Autodesk Inventor part; units mm, degrees
ref_plane "YZ Plane" through (0, 0, 0) normal (1, 0, 0) x (0, 1, 0)
ref_plane "XZ Plane" through (0, 0, 0) normal (0, 1, 0) x (-1, 0, 0)
ref_plane "XY Plane" through (0, 0, 0) normal (0, 0, 1) x (1, 0, 0)
sketch "Sketch10" plane through (0, 0, 0) normal (1, 0, 0) x (0, 1, 0)
  line L0 (0, 0) -> (175, 0)
  line L1 (350, -175) -> (350, -175)
  line L2 (175, -350) -> (0, -350)
  line L3 (0, -350) -> (0, 0)
  arc A0 (350, -175) -> (175, 0) centre (175, -175) ccw
  arc A1 (175, -350) -> (350, -175) centre (175, -175) ccw
  point P0 (350, -350)
  point P1 (350, 0)
  dimension "d73" = 350
  dimension "d74" = 350
  dimension "d76" = 175
extrude "Extrusion19" add sketch "Sketch10" along normal blind 300
sketch "Sketch11" plane through (300, 0, 0) normal (1, 0, 0) x (0, 0, -1)
  arc A0 (350, 175) -> (0, 175) centre (175, 175) ccw
  circle A1 centre (175, 175) radius 60
  point P0 (0, 0)
  dimension "d79" = 120
extrude "Extrusion20" cut sketch "Sketch11" against normal blind 300
sketch "Sketch12" plane through (0, 0, -350) normal (0, -1, 0) x (1, 0, 0)
  line L0 (300, 0) -> (300, 350)
  line L1 (0, 350) -> (300, 350)
  line L2 (300, 350) -> (300, 0)
  line L3 (300, 0) -> (0, 0)
  line L4 (0, 0) -> (0, 350)
extrude "Extrusion21" add sketch "Sketch12" along normal blind 700
sketch "Sketch13" plane through (300, 0, 0) normal (1, 0, 0) x (0, 0, -1)
  circle A0 centre (175, 175) radius 60
  arc A1 (350, 175) -> (0, 175) centre (175, 175) ccw
  arc A2 (350, 175) -> (0, 175) centre (175, 175) ccw
  line L0 (350, 175) -> (350, 0)
  line L1 (350, 0) -> (0, 0)
  line L2 (0, 0) -> (0, 175)
  circle A3 centre (175, 175) radius 60
extrude "Extrusion22" add sketch "Sketch13" along normal blind 150
properties part number "Molde" material "Aluminum 6061"
Can you work these out from the model? Positions are in its coordinate system, mm. A direction names the side the tool comes from. Give positions to 0.01 mm unless a question says otherwise; leave off trailing zeros. Order: outer loops, then holes, each group sorted by start corner. A loop starts at its lowest first (then second) coordinate and runs counter-clockwise, first axis right, second up. Notation, with made-up numbers: M -36.5,43.25 L 22.5,43.25 A19 cw 22.5,76.25 Z; hole C 73,35.5 d8. An arc over 180 degrees is marked long. Write item = value, one per line. Start each with the question number.
Q1. Suppose I cut it at C-C (y = 187.5). Write out the boundary of the cut face in (x, z).
Q2. Will these pins go through, and if not, where does the flat tip stop? pin 1 Ø2 at (x, z) = (144, -104.5) entering from +Y; pin 2 Ø12 at (y, z) = (-503.5, -207.5) entering from +X; pin 3 Ø10 at (y, z) = (-394, -297.5) entering from -X.
Q3. Suppose I cut it at A-A (z = -175). Write out the boundary of the cut face in (x, y), plus the area to 4 significant figures.
Q4. For faces 1 (the flat face through (450, 100, -173)), 2 (the flat face through (374, 0, -177)), which set-ups out of +Z, -Z, +X, -X, +Y, -Y let a thin tool reach every point of the face, with its end or its side?
Q5. I need wall thicknesses on probe 1 along Y at (x, z) = (94, -175); probe 2 along Y at (x, z) = (351, -175); probe 3 along X at (y, z) = (-565, -86.5). Which ranges of each line are inside material? Lowest first, please. Write a range as [from, to].
Q6. Suppose I cut it at D-D (x = 423.5). Write out the boundary of the cut face in (y, z).
Q7. We'd pull the mould along Z, two halves only. Please class faces 3 (the flat face through (300, -345, -177)), 4 (the flat face through (172, -269, 0)), 5 (the cylindrical face through (221.85, 134.449, -130.778)): pulls with the +Z half, pulls with the -Z half, needs draft (parallel to the pull), parting line crosses it, or undercut.
Q8. Suppose I cut it at B-B (x = 36). Write out the boundary of the cut face in (y, z), plus the area to 3 significant figures.
Check result:
q1.outline = M 0,-349.55 L 450,-349.55 L 450,-233.68 L 0,-233.68 Z; M 0,-116.32 L 450,-116.32 L 450,-0.45 L 0,-0.45 Z
q2.pin_1 = 335.61
q2.pin_2 = 300
q2.pin_3 = 0
q3.outline = M 0,-700 L 300,-700 L 300,0 L 450,0 L 450,115 L 0,115 Z; M 0,235 L 450,235 L 450,350 L 0,350 Z
q3.area = 313,500 mm2
q4.face_1 = +Z, -Z, +X, +Y, -Y
q4.face_2 = +Z, -Z, +X, -Y
q5.probe_1 = [-700, 115], [235, 350]
q5.probe_2 = [0, 115], [235, 350]
q5.probe_3 = [0, 300]
q6.outline = M 0,-350 L 175,-350 A175 ccw 175,0 L 0,0 Z; hole C 175,-175 d120
q7.face_3 = needs draft
q7.face_4 = pulls with the +Z half
q7.face_5 = undercut
q8.outline = M -700,-350 L 175,-350 A175 ccw 175,0 L -700,0 Z; hole C 175,-175 d120
q8.area = 343,000 mm2
